from build123d import *

# Parameters (mm, degrees)
BOSS_EXTRUDE1_DEPTH         = 6.35
F_3_4_0_75_DIAMETER_HOLE1_D = 19.05
F_10_0_10_DIAMETER_HOLE1_D  = 10
F_5_8_DIAMETER_HOLE2_D      = 15.875
CUT_EXTRUDE1_REACH          = 205.594
FILLET1_R                   = 35
FILLET3_R                   = 35
FILLET4_R                   = 20
FILLET6_R                   = 40
SKETCH22_R                  = 2.65
CUT_EXTRUDE2_DEPTH          = 10
SKETCH24_R                  = 2.65
CUT_EXTRUDE3_DEPTH          = 10
BOSS_EXTRUDE4_DEPTH         = 6.35
BOSS_EXTRUDE5_DEPTH         = 6.35
SKETCH30_R                  = 2.65
CUT_EXTRUDE4_DEPTH          = 6.35
SKETCH31_R                  = 2.131200652
CUT_EXTRUDE5_DEPTH          = 6.35
SKETCH32_R                  = 2.65
CUT_EXTRUDE6_DEPTH          = 6.35
SKETCH33_R                  = 2.65
SKETCH33_R_2                = 3.724628158
BOSS_EXTRUDE6_DEPTH         = 6.3
CUT_EXTRUDE7_START          = -10
SKETCH34_R                  = 2.65
CUT_EXTRUDE7_DEPTH          = 10
BOSS_EXTRUDE7_START         = -6.3
SKETCH35_R                  = 2.65
BOSS_EXTRUDE7_DEPTH         = 6.3


with BuildPart() as part:
    # Sketch1 → Boss-Extrude1 (new body)
    with BuildSketch(Plane(origin=(0, 0, 0), x_dir=(0, 0, -1), z_dir=(1, 0, 0))):
        with BuildLine():
            Line((-60.717143143, 0), (60.717143143, 0))
            ThreePointArc((60.717143143, 0), (94.584407895, 9.944020783), (67.452353804, 32.521151068))
            Line((67.452353804, 32.521151068), (-134.404938559, 119.878311848))
            ThreePointArc((-134.404938559, 119.878311848), (-155.966181949, 122.347168224), (-149.752887031, 101.553480851))
            Line((-149.752887031, 101.553480851), (-94.55805454, 18.181208272))
            ThreePointArc((-94.55805454, 18.181208272), (-84.465516954, -3.618285637), (-60.717143143, 0))
        make_face()
    extrude(amount=BOSS_EXTRUDE1_DEPTH)

    # 3/4 (0.75) Diameter Hole1 (through all)
    with Locations(Plane(origin=(6.35, 0, 0), x_dir=(0, 0, -1), z_dir=(1, 0, 0))):
        with Locations((75, 14)):
            Hole(F_3_4_0_75_DIAMETER_HOLE1_D / 2)

    # Ø10.0 (10) Diameter Hole1 (through all)
    with Locations(Plane(origin=(6.35, 0, 0), x_dir=(0, 0, -1), z_dir=(1, 0, 0))):
        with Locations((-146, 114)):
            Hole(F_10_0_10_DIAMETER_HOLE1_D / 2)

    # Ø5/8" Diameter Hole2 (through all)
    with Locations(Plane(origin=(6.35, 0, 0), x_dir=(0, 0, -1), z_dir=(1, 0, 0))):
        with Locations((-75, 14)):
            Hole(F_5_8_DIAMETER_HOLE2_D / 2)

    # Sketch8 → Cut-Extrude1 (cut, up to next)
    with BuildSketch(Plane(origin=(6.35, 0, 0), x_dir=(0, 0, -1), z_dir=(1, 0, 0)), mode=Mode.PRIVATE) as cut_extrude1_sk1:
        with BuildLine():
            Line((-52.98768213, 32.027989609), (-48.791838571, 52.287736349))
            ThreePointArc((-48.791838571, 52.287736349), (-43.609219792, 59.133963583), (-35.027937054, 59.43719837))
            Line((-35.027937054, 59.43719837), (22.864909862, 34.383088722))
            ThreePointArc((22.864909862, 34.383088722), (27.230289645, 25.979007794), (19.886136685, 20))
            Line((19.886136685, 20), (-43.195478183, 20))
            ThreePointArc((-43.195478183, 20), (-50.950473221, 23.686518238), (-52.98768213, 32.027989609))
        make_face()
    cut_extrude1_tool1 = extrude(cut_extrude1_sk1.sketch, amount=-CUT_EXTRUDE1_REACH, mode=Mode.PRIVATE) & part.part
    # Sketch8 → Cut-Extrude1 (cut, up to next)
    with BuildSketch(Plane(origin=(6.35, 0, 0), x_dir=(0, 0, -1), z_dir=(1, 0, 0)), mode=Mode.PRIVATE) as cut_extrude1_sk2:
        with BuildLine():
            Line((-75.95726339, 42.34340423), (-63.166421785, 57.61515284))
            ThreePointArc((-63.166421785, 57.61515284), (-61.101947711, 66.340863059), (-66.861018022, 73.213503103))
            Line((-66.861018022, 73.213503103), (-119.037006728, 95.793545572))
            ThreePointArc((-119.037006728, 95.793545572), (-123.11030371, 94.828752024), (-123.345509052, 90.649367698))
            Line((-123.345509052, 90.649367698), (-91.961866267, 43.244103424))
            ThreePointArc((-91.961866267, 43.244103424), (-84.185443207, 38.780101137), (-75.95726339, 42.34340423))
        make_face()
    cut_extrude1_tool2 = extrude(cut_extrude1_sk2.sketch, amount=-CUT_EXTRUDE1_REACH, mode=Mode.PRIVATE) & part.part
    add(cut_extrude1_tool1.solids().sort_by_distance((6.35, 35.497015, 18.727672))[0], mode=Mode.SUBTRACT)
    add(cut_extrude1_tool2.solids().sort_by_distance((6.35, 67.079595, 89.97893))[0], mode=Mode.SUBTRACT)

    # Fillet1
    fillet1_edges = [part.edges().sort_by_distance(p)[0] for p in [
        (3.175, 18.181208272, 94.55805454),
    ]]
    fillet(fillet1_edges, radius=FILLET1_R)

    # Fillet3
    fillet3_edges = [part.edges().sort_by_distance(p)[0] for p in [
        (3.175, 32.521151068, -67.452353804),
        (3.175, 0, -60.717143143),
    ]]
    fillet(fillet3_edges, radius=FILLET3_R)

    # Fillet4
    fillet4_edges = [part.edges().sort_by_distance(p)[0] for p in [
        (3.175, 101.553480851, 149.752887031),
        (3.175, 119.878311848, 134.404938559),
    ]]
    fillet(fillet4_edges, radius=FILLET4_R)

    # Fillet6
    fillet6_edges = [part.edges().sort_by_distance(p)[0] for p in [
        (3.175, 0, 60.717143143),
    ]]
    fillet(fillet6_edges, radius=FILLET6_R)

    # Sketch22 → Cut-Extrude2 (cut)
    with BuildSketch(Plane(origin=(6.35, 0, 0), x_dir=(0, 0, -1), z_dir=(1, 0, 0))):
        with Locations((60.644779113, 26.750227475)):
            Circle(SKETCH22_R)
    extrude(amount=-CUT_EXTRUDE2_DEPTH, mode=Mode.SUBTRACT)

    # Sketch24 → Cut-Extrude3 (cut)
    with BuildSketch(Plane(origin=(6.35, 0, 0), x_dir=(0, 0, -1), z_dir=(1, 0, 0))):
        with Locations((42.966527297, 34.400790246)):
            Circle(SKETCH24_R)
    extrude(amount=-CUT_EXTRUDE3_DEPTH, mode=Mode.SUBTRACT)

    # Sketch25 → Boss-Extrude4 (add)
    with BuildSketch(Plane(origin=(6.35, 0, 0), x_dir=(0, 0, -1), z_dir=(1, 0, 0))):
        with BuildLine():
            ThreePointArc((43.711860671, 42.795251406), (46.681302599, 44.337685596), (48.793885353, 41.74275155))
            ThreePointArc((48.793885353, 41.74275155), (48.738819399, 41.205334304), (48.575910035, 40.690251694))
            Line((48.575910035, 40.690251694), (50.945207618, 39.664898052))
            ThreePointArc((50.945207618, 39.664898052), (48.221738851, 46.544073815), (41.342563089, 43.820605048))
            Line((41.342563089, 43.820605048), (43.711860671, 42.795251406))
        make_face()
    extrude(amount=-BOSS_EXTRUDE4_DEPTH)

    # Sketch29 → Boss-Extrude5 (add)
    with BuildSketch(Plane(origin=(6.35, 0, 0), x_dir=(0, 0, -1), z_dir=(1, 0, 0))):
        with BuildLine():
            ThreePointArc((69.263055818, 33.964695583), (65.196576348, 39.805321361), (59.068365536, 36.186730888))
            ThreePointArc((59.068365536, 36.186730888), (60.5303447, 35.66620465), (62.013960909, 35.210997462))
            ThreePointArc((62.013960909, 35.210997462), (64.343055459, 36.809883075), (66.21463271, 34.693680056))
            ThreePointArc((66.21463271, 34.693680056), (66.205602012, 34.497647468), (66.178586414, 34.303275437))
            ThreePointArc((66.178586414, 34.303275437), (67.717067085, 34.099786208), (69.263055818, 33.964695583))
        make_face()
    extrude(amount=-BOSS_EXTRUDE5_DEPTH)

    # Sketch30 → Cut-Extrude4 (cut)
    with BuildSketch(Plane(origin=(6.35, 0, 0), x_dir=(0, 0, -1), z_dir=(1, 0, 0))):
        with Locations((46.143885353, 41.74275155)):
            Circle(SKETCH30_R)
    extrude(amount=-CUT_EXTRUDE4_DEPTH, mode=Mode.SUBTRACT)

    # Sketch31 → Cut-Extrude5 (cut)
    with BuildSketch(Plane(origin=(6.35, 0, 0), x_dir=(0, 0, -1), z_dir=(1, 0, 0))):
        with Locations((64.096273662, 34.757136449)):
            Circle(SKETCH31_R)
    extrude(amount=-CUT_EXTRUDE5_DEPTH, mode=Mode.SUBTRACT)

    # Sketch32 → Cut-Extrude6 (cut)
    with BuildSketch(Plane(origin=(6.35, 0, 0), x_dir=(0, 0, -1), z_dir=(1, 0, 0))):
        with Locations((64.096273662, 34.757136449)):
            Circle(SKETCH32_R)
    extrude(amount=-CUT_EXTRUDE6_DEPTH, mode=Mode.SUBTRACT)

    # Sketch33 → Boss-Extrude6 (add)
    with BuildSketch(Plane(origin=(6.35, 0, 0), x_dir=(0, 0, -1), z_dir=(1, 0, 0))):
        with Locations((42.966527297, 34.400790246)):
            Circle(SKETCH33_R)
        with Locations((60.715336282, 26.683263033)):
            Circle(SKETCH33_R_2)
    extrude(amount=-BOSS_EXTRUDE6_DEPTH)

    # Sketch34 → Cut-Extrude7 (cut)
    with BuildSketch(Plane.ZY.offset(CUT_EXTRUDE7_START)):
        with Locations(Location((-60.644779113, 26.750227475, 0), (0, 0, 180))):
            Circle(SKETCH34_R)
        with Locations(Location((-42.966527297, 34.400790246, 0), (0, 0, 180))):
            Circle(SKETCH34_R)
    extrude(amount=CUT_EXTRUDE7_DEPTH, mode=Mode.SUBTRACT)

    # Sketch35 → Boss-Extrude7 (add)
    with BuildSketch(Plane.ZY.offset(BOSS_EXTRUDE7_START)):
        with Locations(Location((-60.644779113, 26.750227475, 0), (0, 0, 180))):
            Circle(SKETCH35_R)
        with Locations(Location((-42.966527297, 34.400790246, 0), (0, 0, 180))):
            Circle(SKETCH35_R)
    extrude(amount=BOSS_EXTRUDE7_DEPTH)


solid = part.part
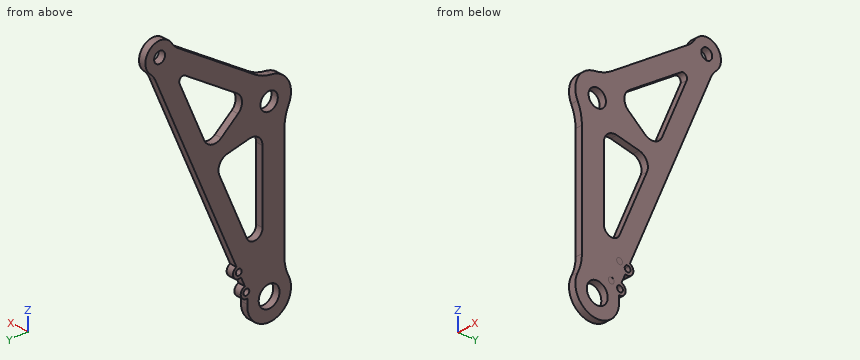
Build history of the part. All positions in model axes, mm. Round coordinates to 2 decimals unless told otherwise and drop trailing zeros. Write each loop counter-clockwise with the first axis right and the second up, starting at its lowest first coordinate (ties: lowest second). Pieces come first, ordered by that corner, then holes. Notation, with made-up numbers: (5, 8) - (49, 8) arc R17 ccw to (49, 29) - close; hole circle Ø2 at (89.5, -23.75). An arc over 180 degrees is marked (long way). Use CSV: the item, a comma, the result in double quotes.
(1) Band-saw the part on B-B (z = 3.5). Write the cut outline in (x, y), plus the area to 3 significant figures.
Response:
outline,"(0, 0) - (6.35, 0) - (6.35, 20) - (0, 20) - close; (0, 45.79) - (6.35, 45.79) - (6.35, 63.23) - (0, 63.23) - close"
area,"238 mm²"
(2) Band-saw the part on C-C (x = 1). Give the number of separate pieces and of enclosed holes in the cut face, plus the area to 3 significant figures.
Response:
separate pieces,"1"
enclosed holes,"7"
area,"10,800 mm²"
(3) Band-saw the part on A-A (y = 86.5). Write the cut outline in (x, z), plus the area to 3 significant figures.
Response:
outline,"(0, 57.28) - (6.35, 57.28) - (6.35, 97.56) - (0, 97.56) - close; (0, 120.6) - (6.35, 120.6) - (6.35, 139.79) - (0, 139.79) - close"
area,"378 mm²"
(4) Pin check, flat tips, straight feed: P1, Ø1.5, axis at x = 4, z = -33.5, coming from the +Y side; P2, Ø1, axis at x = 2, y = 93, coming from the +Z side; P3, Ø1.6, axis at y = 33.5, z = -44, coming from the +X side. Stop position of each tip, or through.
Response:
P1,"y = 47.54"
P2,"z = 144.42"
P3,"x = 6.3"
(5) Wall check: line 1 (Z direction, x = 1, y = 18); line 2 (Z direction, x = 2.25, y = 47.5); line 3 (Z direction, x = 1, y = 21) (3 decimals). Give the ranges that are in metal, low to high.
Response:
line 1,"-94.6 to -83.64, -66.36 to 68.14, 81.86 to 96.17"
line 2,"-32.84 to 7.44, 49.78 to 71.64, 94.78 to 113.97"
line 3,"-93.735 to -81.46, -68.54 to -23.628, 47.554 to 71.258, 78.742 to 97.24"
